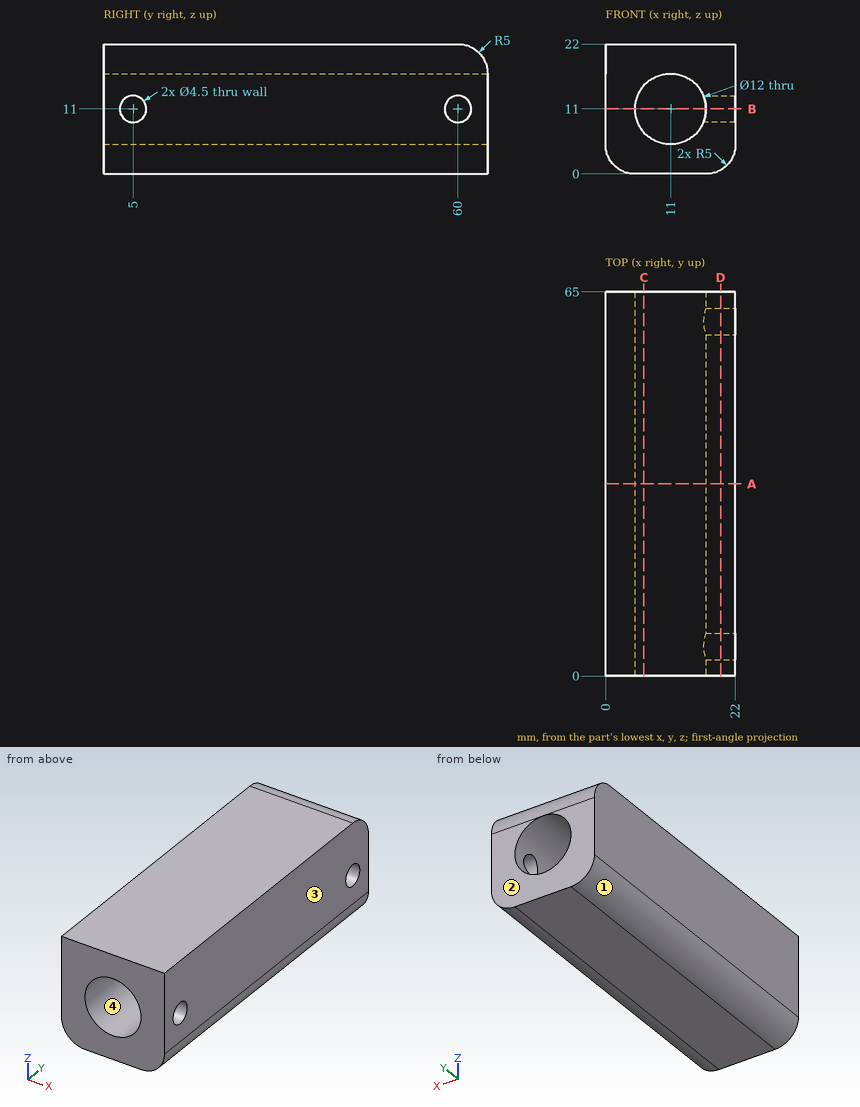
For this review, use the dimensioned drawing (mm, ordinates from the lowest corner) and the shaded views. Coordinates: 2 decimals unless noted, no trailing zeros. Order: outer loops, then holes, each group sorted by start corner. A loop starts at its lowest first (then second) coordinate and runs counter-clockwise, first axis right, second up. Notation, with made-up numbers: (86.5, -9.75) - (120.5, -9.75) arc R16 cw to (120.5, 13.25) - close; hole circle Ø4 at (71.5, -12). An arc over 180 degrees is marked (long way). Answer as a JSON object with one key per item and string values. Group by question number.
1. The part is to be moulded in two halves that separate along X. For the marked faces 1, 2, 3 and 4, say which applies: pulls with the +X half, pulls with the -X half, needs draft (parallel to the pull), parting line crosses it, or undercut.
2. Clearance check with flat-ended pins moving along their axes: P1, Ø5, axis at x = 4, y = 31.5, coming from the -Z side; P2, Ø3.5, axis at y = 60, z = 11, coming from the +X side; P3, Ø2.5, axis at y = 5, z = 11, coming from the +X side. State where each tip first meets the part, or that it passes through.
3. We need section C-C on x = 6.5. State the section outline as (y, z) points.
4. We need section B-B on z = 11. State the section outline as (x, y) points, then the cut area to 3 significant figures.
5. For probe 1 along Y at (x, z) = (20.35, 11); probe 2 along X at (y, z) = (46, 11); probe 3 along X at (y, z) = (35, 6.5), list the stretches that pass through material, from the lowest coordinate up.
6. We need section D-D on x = 19.5. State the section outline as (y, z) points.
7. We need section A-A on y = 32.5. State the section outline as (x, z) points, then the cut area to 3 significant figures.
Final values:
{
 "1": {"face 1": "pulls with the -X half", "face 2": "needs draft", "face 3": "pulls with the +X half", "face 4": "undercut"},
 "2": {"P1": "z = 0", "P2": "x = 5.26", "P3": "x = 5.13"},
 "3": {"outline": "(0, 0) - (65, 0) - (65, 7.03) - (0, 7.03) - close; (0, 14.97) - (65, 14.97) - (65, 17) arc R5 ccw to (60, 22) - (0, 22) - close"},
 "4": {"outline": "(0, 0) - (5, 0) - (5, 65) - (0, 65) - close; (17, 0) - (22, 0) - (22, 2.75) - (17, 2.75) - close; (17, 7.25) - (22, 7.25) - (22, 57.75) - (17, 57.75) - close; (17, 62.25) - (22, 62.25) - (22, 65) - (17, 65) - close", "area": "605 mm²"},
 "5": {"probe 1": "0 to 2.75, 7.25 to 57.75, 62.25 to 65", "probe 2": "0 to 5, 17 to 22", "probe 3": "0 to 7.03, 14.97 to 22"},
 "6": {"outline": "(0, 0.67) - (65, 0.67) - (65, 17) arc R5 ccw to (60, 22) - (0, 22) - close; hole circle Ø4.5 at (5, 11); hole circle Ø4.5 at (60, 11)"},
 "7": {"outline": "(0, 5) arc R5 ccw to (5, 0) - (17, 0) arc R5 ccw to (22, 5) - (22, 22) - (0, 22) - close; hole circle Ø12 at (11, 11)", "area": "360 mm²"}
}
